Input: part model. Units: mm. Frame: model coordinates. A direction names the side the tool comes from. Round coordinates to 2 decimals unless told otherwise and drop trailing zeros. Write each loop counter-clockwise with the first axis right and the second up, starting at its lowest first coordinate (ties: lowest second). Pieces come first, ordered by that corner, then holes. Notation, with made-up numbers: (44.5, 34) -> (91.5, 34) arc R15 ccw to (91.5, 38) -> close; hole circle Ø9 at (58, 60). An arc over 180 degrees is marked (long way). Write item = value, one per line. Start each with the question number.
```python
from build123d import *

# Parameters (mm, degrees)
F0_W          = 58.8852874935
F0_H          = 62.7336800098
F1_DEPTH      = 63.5
F2_W          = 65.9335851669
F2_H          = 13.4996175766
F3_DEPTH      = 30.1423424313
F3_DEPTH_BACK = 28.7439450622
F4_R          = 5.08
F5_R          = 5.08
F6_R          = 5.08
F7_W          = 35.6836467981
F7_H          = 28.7272408605
F8_DEPTH      = 25.4
F10_D         = 25.4


with BuildPart() as f1:
    # F0 (on Front) → F1 (new body, symmetric)
    with BuildSketch(Plane.XZ):
        with Locations((0.6986986846, 2.6395991445)):
            Rectangle(F0_W, F0_H)
    extrude(amount=F1_DEPTH, both=True)

    # F2 (on Right) → F3 (cut, two sides)
    with BuildSketch(Plane.YZ) as f3_sk:
        with Locations((-1.4819055796, 6.7498087883)):
            Rectangle(F2_W, F2_H)
    extrude(amount=F3_DEPTH, mode=Mode.SUBTRACT)
    extrude(f3_sk.sketch, amount=-F3_DEPTH_BACK, mode=Mode.SUBTRACT)

    # F4
    f4_edges = [f1.edges().sort_by_distance(p)[0] for p in [
        (0.698699, 63.5, 34.006439),
    ]]
    fillet(f4_edges, radius=F4_R)

    # F5
    f5_edges = [f1.edges().sort_by_distance(p)[0] for p in [
        (0.698699, -63.5, 34.006439),
    ]]
    fillet(f5_edges, radius=F5_R)

    # F6
    f6_edges = [f1.edges().sort_by_distance(p)[0] for p in [
        (-28.743945, 0, -28.727241),
        (-28.743945, -63.5, 0.099599),
        (-28.743945, 63.5, 0.099599),
        (30.141342, 63.5, 0.099599),
        (30.141342, 0, 34.006439),
        (-28.743945, 0, 34.006439),
        (0.698699, 63.5, -28.727241),
    ]]
    fillet(f6_edges, radius=F6_R)

    # F7 (on face) → F8 (join)
    with BuildSketch(Plane.YZ.offset(30.1413424313)):
        with Locations((-0.0774413347, -14.3636204302)):
            Rectangle(F7_W, F7_H)
    extrude(amount=F8_DEPTH)

    # F10 (through all)
    with Locations(Plane.XY.offset(34.0064391494)):
        with Locations((0, 0)):
            Hole(F10_D / 2)


solid = f1.part
```
1. Reachability of faces 4 (the flat face through (0, -14, 34.006)), 5 (the flat face through (43, 17.764, -15)), 6 (the flat face through (14, -2, 0)) from +Z, -Z, +X, -X, +Y, -Y: full face, straight path, thin tool, end or side. Return the list, or none.
2. Pin query (flat end, axial travel): P1, Ø20.5, axis at x = 0, y = 0, coming from the -Z side; P2, Ø8, axis at y = -46, z = -19.5, coming from the +X side; P3, Ø12.5, axis at x = 47, z = -12, coming from the +Y side. Return the tip coordinate at first contact, or that it passes through.
3. Section D-D (y = -24). Output: boundary loops of the cut face in (x, z).
4. Section A-A (z = 12). Output: boundary loops of the cut face in (x, y).
5. Line query: line 1 along Y through (x, z) = (0, -10.75); line 2 along Y through (x, z) = (-21.5, 0.5); line 3 along Z through (x, y) = (5, -15). Output: solid intervals per line, ascending.
6. Section C-C (x = 0). Output: boundary loops of the cut face in (y, z).
7. Section B-B (y = 0). Output: boundary loops of the cut face in (x, z), then the cut area to 3 significant figures.
8. Mould query, pull axis X, two halves, no side actions, for faces 1 (the cylindrical face through (2.75, -12.4, -14.56)), 2 (the cylindrical face through (-27.3, 61.97, 2.27)), 3 (the cylindrical face through (28.61, -0.82, 32.56)). Classes: pulls with the +X half, pulls with the -X half, needs draft (parallel to the pull), parting line crosses it, or undercut.
Check sheet entries:
q1.face_4 = +Z, +X, -X, +Y, -Y
q1.face_5 = +Z, -Z, +X, +Y
q1.face_6 = +X, -X
q2.P1 = through
q2.P2 = 30.14
q2.P3 = 17.76
q3.outline = (-28.74, -23.65) arc R5.08 ccw to (-23.66, -28.73) -> (30.14, -28.73) -> (30.14, 0) -> (-28.74, 0) -> close; (-28.74, 13.5) -> (30.14, 13.5) -> (30.14, 28.93) arc R5.08 ccw to (25.06, 34.01) -> (-23.66, 34.01) arc R5.08 ccw to (-28.74, 28.93) -> close
q4.outline = (-28.74, -58.42) arc R5.08 ccw to (-23.66, -63.5) -> (25.06, -63.5) arc R5.08 ccw to (30.14, -58.42) -> (30.14, -34.45) -> (-28.74, -34.45) -> close; (-28.74, 31.48) -> (30.14, 31.48) -> (30.14, 58.42) arc R5.08 ccw to (25.06, 63.5) -> (-23.66, 63.5) arc R5.08 ccw to (-28.74, 58.42) -> close
q5.line_1 = -63.5 to -12.7, 12.7 to 63.5
q5.line_2 = -63.5 to -34.45, 31.48 to 63.5
q5.line_3 = -28.73 to 0, 13.5 to 34.01
q6.outline = (-63.5, -28.73) -> (-12.7, -28.73) -> (-12.7, 0) -> (-34.45, 0) -> (-34.45, 13.5) -> (-12.7, 13.5) -> (-12.7, 34.01) -> (-58.42, 34.01) arc R5.08 ccw to (-63.5, 28.93) -> close; (12.7, -28.73) -> (58.42, -28.73) arc R5.08 ccw to (63.5, -23.65) -> (63.5, 28.93) arc R5.08 ccw to (58.42, 34.01) -> (12.7, 34.01) -> (12.7, 13.5) -> (31.48, 13.5) -> (31.48, 0) -> (12.7, 0) -> close
q7.outline = (-28.74, -23.65) arc R5.08 ccw to (-23.66, -28.73) -> (-12.7, -28.73) -> (-12.7, 0) -> (-28.74, 0) -> close; (-28.74, 13.5) -> (-12.7, 13.5) -> (-12.7, 34.01) -> (-23.66, 34.01) arc R5.08 ccw to (-28.74, 28.93) -> close; (12.7, -28.73) -> (55.54, -28.73) -> (55.54, 0) -> (12.7, 0) -> close; (12.7, 13.5) -> (30.14, 13.5) -> (30.14, 28.93) arc R5.08 ccw to (25.06, 34.01) -> (12.7, 34.01) -> close
q7.area = 2,360 mm2
q8.face_1 = undercut
q8.face_2 = pulls with the -X half
q8.face_3 = pulls with the +X half
